Can you work these out from the model? Positions are in its coordinate system, mm. A direction names the side the tool comes from. Round coordinates to 2 decimals unless told otherwise and drop trailing zeros. Loops run counter-clockwise (first coordinate to the right, second up) from the corner with the lowest first, then second, coordinate; pieces in that order, holes last.
(1) Will these pins go through, and if not, where does the flat tip stop? pin 1 Ø12 at (x, z) = (36.5, 45) entering from +Y; pin 2 Ø2 at (x, z) = (26, 35) entering from -Y; pin 3 Ø2 at (x, y) = (41, -3.5) entering from +Z.
(2) Which directions (+Z, -Z, +X, -X, +Y, -Y) give clear straight access to the entire face, cutting with the end or side of a thin tool? Please do faces 5 (the face through (34.83, -0.75, 22.97)), 6 (the face through (34.825, 1.362, 22.333)), 7 (the face through (-20.5, 0, 38)), 8 (the face through (35, -4, 45.301)).
(3) I want a section at B-B on x = 41. Write out the boundary of the cut face in (y, z).
(4) I want a section at C-C on z = 29. Give the number of separate pieces and of enclosed holes in the cut face, plus the area to 3 significant figures.
(5) Thinking about a two-plate mould opening in Y: for faces 1 (the face through (41.95, -1.1, 30.71)), 2 (the face through (19, -11.57, 37.96)), 3 (the face through (21.07, 13.5, 34.51)), 4 (the face through (-1.8, 13.4, 70)), which applies, released by +Y, released by -Y, zero draft, split by the parting line, or undercut?
(6) I want a section at D-D on x = 12. Write out the boundary of the cut face in (y, z).
(7) I want a section at A-A on z = 50. Write out the boundary of the cut face in (x, y), plus the area to 3 significant figures.
(8) If I drill on line 1 along Y through (x, z) = (-2, 60); line 2 along X through (y, z) = (-2.5, 47.5); line 3 along Z through (x, y) = (-10.5, -5.5), over which ranges is the centre line in solid material (lowest first)?
from build123d import *

# Parameters (mm, degrees)
PAD_DEPTH       = 70
POCKET_DEPTH    = 65
PAD001_DEPTH    = 25
SKETCH003_R     = 7.5
POCKET001_DEPTH = 5


with BuildPart() as part:
    # Sketch → Pad (new body)
    with BuildSketch(Plane.XY):
        with BuildLine():
            Line((-22.5, 10), (-22.5, -10))
            ThreePointArc((-22.5, -10), (-21.035534, -13.535534), (-17.5, -15))
            Line((-17.5, -15), (17.5, -15))
            ThreePointArc((17.5, -15), (21.035534, -13.535534), (22.5, -10))
            Line((22.5, -10), (22.5, 10))
            ThreePointArc((22.5, 10), (21.035534, 13.535534), (17.5, 15))
            Line((17.5, 15), (-17.5, 15))
            ThreePointArc((-17.5, 15), (-21.035534, 13.535534), (-22.5, 10))
        make_face()
    extrude(amount=PAD_DEPTH)

    # Sketch001 (on Face10 of Pad) → Pocket (cut)
    with BuildSketch(Plane.XY.offset(70)):
        with BuildLine():
            Line((-20.5, 8), (-20.5, -8))
            ThreePointArc((-20.5, -8), (-19.035534, -11.535534), (-15.5, -13))
            Line((-15.5, -13), (15.5, -13))
            ThreePointArc((15.5, -13), (19.035534, -11.535534), (20.5, -8))
            Line((20.5, -8), (20.5, 8))
            ThreePointArc((20.5, 8), (19.035534, 11.535534), (15.5, 13))
            Line((15.5, 13), (-15.5, 13))
            ThreePointArc((-15.5, 13), (-19.035534, 11.535534), (-20.5, 8))
        make_face()
    extrude(amount=-POCKET_DEPTH, mode=Mode.SUBTRACT)

    # Sketch002 (on Face9 of Pocket) → Pad001 (join)
    with BuildSketch(Plane.YZ.offset(22.5)):
        Polygon((5.3, 0), (-2.687816, 45.301157), (-4.687816, 45.301157), (3.3, 0), align=None)
    extrude(amount=PAD001_DEPTH)

    # Sketch003 (on Face20 of Pad001) → Pocket001 (cut)
    with BuildSketch(Plane(origin=(0, 5.140185, 0.906353), x_dir=(-1, 0, 0), z_dir=(0, 0.984808, 0.173648))):
        with Locations((-36, 35)):
            Circle(SKETCH003_R)
        with Locations((-36, 12)):
            Circle(SKETCH003_R)
    extrude(amount=-POCKET001_DEPTH, mode=Mode.SUBTRACT)


solid = part.part
Filled sheet:
1. pin 1: stops at y = -1.92
1. pin 2: stops at y = -3.05
1. pin 3: stops at z = 45.3
2. face 5: -Z, +X, -Y
2. face 6: +Z, +X, +Y
2. face 7: +Z
2. face 8: +Z, +X, +Y, -Y
3. outline: (-4.69, 45.3) - (-3.85, 40.54) - (-1.91, 40.88) - (-2.69, 45.3) - close; (-1.91, 29.53) - (0.15, 17.89) - (2.09, 18.23) - (0.03, 29.87) - close; (2.09, 6.88) - (3.3, 0) - (5.3, 0) - (4.03, 7.22) - close
4. separate pieces: 2
4. enclosed holes: 1
4. area: 318 mm2
5. face 1: split by the parting line
5. face 2: undercut
5. face 3: released by +Y
5. face 4: zero draft
6. outline: (-15, 0) - (15, 0) - (15, 70) - (13, 70) - (13, 5) - (-13, 5) - (-13, 70) - (-15, 70) - close
7. outline: (-22.5, -10) arc R5 ccw to (-17.5, -15) - (17.5, -15) arc R5 ccw to (22.5, -10) - (22.5, 10) arc R5 ccw to (17.5, 15) - (-17.5, 15) arc R5 ccw to (-22.5, 10) - close; hole (-20.5, -8) arc R5 ccw to (-15.5, -13) - (15.5, -13) arc R5 ccw to (20.5, -8) - (20.5, 8) arc R5 ccw to (15.5, 13) - (-15.5, 13) arc R5 ccw to (-20.5, 8) - close
7. area: 284 mm2
8. line 1: y = -15 to -13, 13 to 15
8. line 2: x = -22.5 to -20.5, 20.5 to 22.5
8. line 3: z = 0 to 5
